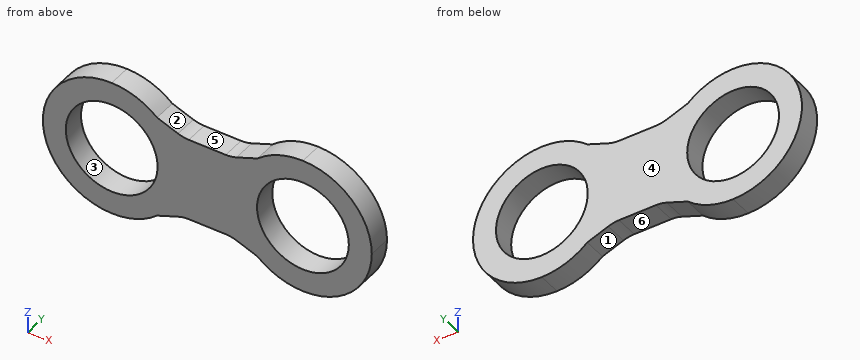
from build123d import *

# Parameters (mm, degrees)
F1_DEPTH = 19.05
F2_R     = 38.1
F3_DEPTH = 25.4


with BuildPart() as f1:
    # F0 (on Front) → F1 (new body)
    with BuildSketch(Plane.XZ):
        with BuildLine():
            Line((20.027097595, 36.4074036121), (2.6105293283, 42.9636023111))
            ThreePointArc((2.6105293283, 42.9636023111), (16.9814393634, 23.5834144733), (22.0743066938, 0))
            ThreePointArc((22.0743066938, 0), (16.9814393634, -23.5834144733), (2.6105293283, -42.9636023111))
            Line((2.6105293283, -42.9636023111), (20.027097595, -36.4074036121))
            ThreePointArc((20.027097595, -36.4074036121), (24.4278254251, -35.189367606), (28.975523916, -34.7789341976))
            Line((28.975523916, -34.7789341976), (59.6230894717, -34.7789341976))
            ThreePointArc((59.6230894717, -34.7789341976), (64.1707879626, -35.189367606), (68.5715157927, -36.4074036121))
            Line((68.5715157927, -36.4074036121), (85.9880840594, -42.9636023111))
            ThreePointArc((85.9880840594, -42.9636023111), (66.5243066938, 0), (85.9880840594, 42.9636023111))
            Line((85.9880840594, 42.9636023111), (68.5715157927, 36.4074036121))
            ThreePointArc((68.5715157927, 36.4074036121), (64.1707879626, 35.189367606), (59.6230894717, 34.7789341976))
            Line((59.6230894717, 34.7789341976), (28.975523916, 34.7789341976))
            ThreePointArc((28.975523916, 34.7789341976), (24.4278254251, 35.189367606), (20.027097595, 36.4074036121))
        make_face()
        with BuildLine():
            ThreePointArc((2.6105293283, 42.9636023111), (-14.941734084, 53.4859438174), (-35.0756933062, 57.15))
            Line((-35.0756933062, 57.15), (2.6105293283, 42.9636023111))
        make_face()
        with BuildLine():
            Line((123.6743066938, 57.15), (85.9880840594, 42.9636023111))
            ThreePointArc((85.9880840594, 42.9636023111), (66.5243066938, 0), (85.9880840594, -42.9636023111))
            Line((85.9880840594, -42.9636023111), (123.6743066938, -57.15))
            ThreePointArc((123.6743066938, -57.15), (164.0854592386, -40.4111525448), (180.8243066938, 0))
            ThreePointArc((180.8243066938, 0), (164.0854592386, 40.4111525448), (123.6743066938, 57.15))
        make_face()
        with BuildLine():
            ThreePointArc((123.6743066938, 57.15), (103.5403474717, 53.4859438174), (85.9880840594, 42.9636023111))
            Line((85.9880840594, 42.9636023111), (123.6743066938, 57.15))
        make_face()
        with BuildLine():
            Line((2.6105293283, 42.9636023111), (-35.0756933062, 57.15))
            ThreePointArc((-35.0756933062, 57.15), (-92.2256933062, 0), (-35.0756933062, -57.15))
            Line((-35.0756933062, -57.15), (2.6105293283, -42.9636023111))
            ThreePointArc((2.6105293283, -42.9636023111), (16.9814393634, -23.5834144733), (22.0743066938, 0))
            ThreePointArc((22.0743066938, 0), (16.9814393634, 23.5834144733), (2.6105293283, 42.9636023111))
        make_face()
        with BuildLine():
            Line((2.6105293283, -42.9636023111), (-35.0756933062, -57.15))
            ThreePointArc((-35.0756933062, -57.15), (-14.941734084, -53.4859438174), (2.6105293283, -42.9636023111))
        make_face()
        with BuildLine():
            Line((123.6743066938, -57.15), (85.9880840594, -42.9636023111))
            ThreePointArc((85.9880840594, -42.9636023111), (103.5403474717, -53.4859438174), (123.6743066938, -57.15))
        make_face()
    extrude(amount=F1_DEPTH)

    # F2 (on face) → F3 (cut)
    with BuildSketch(Plane.XZ.offset(19.05)):
        with Locations((-35.0756933062, 0)):
            Circle(F2_R)
        with Locations((123.6743066938, 0)):
            Circle(F2_R)
    extrude(amount=-F3_DEPTH, mode=Mode.SUBTRACT)


solid = f1.part
The listing builds one solid part. Answer for the finished solid, in the listing's coordinates (mm). Face numbers are marked on the shaded views. A direction names the side the tool comes from. Coordinates: 2 decimals unless noted, no trailing zeros. Write each loop counter-clockwise with the first axis right and the second up, starting at its lowest first coordinate (ties: lowest second). Pieces come first, ordered by that corner, then holes. Notation, with made-up numbers: M 67,1 L 73,1 A25 ccw 73,28 Z; hole C -37.75,-25.5 d10. An arc over 180 degrees is marked long. Put each result on its own line as item: value. Start each with the question number.
1. A cutting plane is placed at C-C on z = 25. Write down the section's boundary in (x, y), then the cut area to 3 significant figures.
2. A cutting plane is placed at B-B on x = 134.5. Write down the section's boundary in (y, z), then the cut area to 3 significant figures.
3. Which of the six approach directions +Z, -Z, +X, -X, +Y, -Y give full straight-line access (tool end or side, diameter ignored) to the marked faces 4, 5 and 6?
4. For a pull along Z with two mould halves and no side action, classify the marked faces 1, 2 and 3 as pulls with the +Z half, pulls with the -Z half, needs draft (parallel to the pull), parting line crosses it, or undercut.
5. A cutting plane is placed at D-D on x = -51.5. Write down the section's boundary in (y, z), then the cut area to 3 significant figures.
6. A cutting plane is placed at A-A on y = -14. Write down the section's boundary in (x, z), then the cut area to 3 significant figures.
7. Consider line 1 (X direction, y = -4.25, z = -1); line 2 (X direction, y = -17.5, z = 34.5); line 3 (Z direction, x = -54, y = -7). Determine where each line is inside the solid, lowest interval first. Write a range as from..to.
8. Flat-ended cylindrical pins translate along their axes: P1, Ø3, axis at x = -54.5, y = -17, coming from the -Z side; P2, Ø10, axis at x = 75, y = -7, coming from the +Z side; P3, Ø9.5, axis at x = 46.5, y = -8.5, coming from the +Z side. Find the tip coordinate at first contact, or state that the pin passes through.
Resolved:
1. outline: M -86.47,-19.05 L -63.83,-19.05 L -63.83,0 L -86.47,0 Z; M -6.32,-19.05 L 94.92,-19.05 L 94.92,0 L -6.32,0 Z; M 152.43,-19.05 L 175.07,-19.05 L 175.07,0 L 152.43,0 Z
1. area: 2,790 mm2
2. outline: M -19.05,-56.12 L 0,-56.12 L 0,-36.53 L -19.05,-36.53 Z; M -19.05,36.53 L 0,36.53 L 0,56.12 L -19.05,56.12 Z
2. area: 746 mm2
3. face 4: +Z, -Z, +X, -X, +Y
3. face 5: +Z, +Y, -Y
3. face 6: -Z, +Y, -Y
4. face 1: pulls with the -Z half
4. face 2: pulls with the +Z half
4. face 3: undercut
5. outline: M -19.05,-54.74 L 0,-54.74 L 0,-34.38 L -19.05,-34.38 Z; M -19.05,34.38 L 0,34.38 L 0,54.74 L -19.05,54.74 Z
5. area: 776 mm2
6. outline: M 2.61,-42.96 L 20.03,-36.41 A25.4 cw 28.98,-34.78 L 59.62,-34.78 A25.4 cw 68.57,-36.41 L 85.99,-42.96 A57.15 ccw long 85.99,42.96 L 68.57,36.41 A25.4 cw 59.62,34.78 L 28.98,34.78 A25.4 cw 20.03,36.41 L 2.61,42.96 A57.15 ccw long Z; hole C -35.08,0 d76.2; hole C 123.67,0 d76.2
6. area: 15,200 mm2
7. line 1: x = -92.22..-73.16, 3.01..85.59, 161.76..180.82
7. line 2: x = -80.64..-51.24, -18.91..107.51, 139.84..169.24
7. line 3: z = -53.93..-33.07, 33.07..53.93
8. P1: stops at z = -54.27
8. P2: stops at z = 40.71
8. P3: stops at z = 34.78
